```python
from build123d import *

# Parameters (mm, degrees)
BOX018_W     = 3.1
BOX018_H     = 1.2
BOX018_DEPTH = 0.2
BOX017_W     = 0.6
BOX017_H     = 1.1
BOX017_DEPTH = 0.2
BOX016_W     = 0.6
BOX016_H     = 1.1
BOX016_DEPTH = 0.2
BOX015_W     = 0.6
BOX015_H     = 1.1
BOX015_DEPTH = 0.2
BOX014_W     = 0.6
BOX014_H     = 1.1
BOX014_DEPTH = 0.2
BOX019_W     = 7.2
BOX019_H     = 3.5
BOX019_DEPTH = 0.2


with BuildPart() as cube018:
    # Box018 → Box018 (new body)
    with BuildSketch(Plane(origin=(2.05, 0, 1.3), x_dir=(1, 0, 0), z_dir=(0, 0, 1))):
        with Locations((1.55, 0.6)):
            Rectangle(BOX018_W, BOX018_H)
    extrude(amount=BOX018_DEPTH)


with BuildPart() as cube017:
    # Box017 → Box017 (new body)
    with BuildSketch(Plane(origin=(0, 2.4, 1.3), x_dir=(1, 0, 0), z_dir=(0, 0, 1))):
        with Locations((0.3, 0.55)):
            Rectangle(BOX017_W, BOX017_H)
    extrude(amount=BOX017_DEPTH)


with BuildPart() as cube016:
    # Box016 → Box016 (new body)
    with BuildSketch(Plane.XY.offset(1.3)):
        with Locations((0.3, 0.55)):
            Rectangle(BOX016_W, BOX016_H)
    extrude(amount=BOX016_DEPTH)


with BuildPart() as cube015:
    # Box015 → Box015 (new body)
    with BuildSketch(Plane(origin=(6.6, 2.4, 1.3), x_dir=(1, 0, 0), z_dir=(0, 0, 1))):
        with Locations((0.3, 0.55)):
            Rectangle(BOX015_W, BOX015_H)
    extrude(amount=BOX015_DEPTH)


with BuildPart() as cube014:
    # Box014 → Box014 (new body)
    with BuildSketch(Plane(origin=(6.6, 0, 1.3), x_dir=(1, 0, 0), z_dir=(0, 0, 1))):
        with Locations((0.3, 0.55)):
            Rectangle(BOX014_W, BOX014_H)
    extrude(amount=BOX014_DEPTH)


with BuildPart() as silver_top:
    # Box019 → Box019 (new body)
    with BuildSketch(Plane.XY.offset(1.3)):
        with Locations((3.6, 1.75)):
            Rectangle(BOX019_W, BOX019_H)
    extrude(amount=BOX019_DEPTH)

    # Cut: cut Cube014
    add(cube014.part, mode=Mode.SUBTRACT)

    # Cut001: cut Cube015
    add(cube015.part, mode=Mode.SUBTRACT)

    # Cut002: cut Cube016
    add(cube016.part, mode=Mode.SUBTRACT)

    # Cut003: cut Cube017
    add(cube017.part, mode=Mode.SUBTRACT)

    # Cut004: cut Cube018
    add(cube018.part, mode=Mode.SUBTRACT)


solid = silver_top.part
```
Check sheet for the modelled part. Datum: model origin and axes. Units: mm. Round coordinates to 2 decimals unless told otherwise and drop trailing zeros. Loops run counter-clockwise (first coordinate to the right, second up) from the corner with the lowest first, then second, coordinate; pieces in that order, holes last. Notation, with made-up numbers: (-40, -21) -> (2, -21) arc R20 cw to (2, -17) -> close; hole circle Ø2 at (-3, 10). An arc over 180 degrees is marked (long way). Write item = value, one per line. Start each with the question number.
1) Sectioned sample at C-C, the plane x = 4.5. Record the cut outline in (y, z), plus the area to 3 significant figures.
2) Sectioned sample at B-B, the plane y = 3.25. Record the cut outline in (x, z).
3) Thickness scan on probe 1 along X at (y, z) = (0.45, 1.45); probe 2 along Y at (x, z) = (0.5, 1.4); probe 3 along X at (y, z) = (2.7, 1.4). Record the ranges inside material, lowest first.
4) Sectioned sample at A-A, the plane z = 1.4. Record the cut outline in (x, y).
Results are:
q1.outline = (1.2, 1.3) -> (3.5, 1.3) -> (3.5, 1.5) -> (1.2, 1.5) -> close
q1.area = 0.460 mm^2
q2.outline = (0.6, 1.3) -> (6.6, 1.3) -> (6.6, 1.5) -> (0.6, 1.5) -> close
q3.probe_1 = 0.6 to 2.05, 5.15 to 6.6
q3.probe_2 = 1.1 to 2.4
q3.probe_3 = 0.6 to 6.6
q4.outline = (0, 1.1) -> (0.6, 1.1) -> (0.6, 0) -> (2.05, 0) -> (2.05, 1.2) -> (5.15, 1.2) -> (5.15, 0) -> (6.6, 0) -> (6.6, 1.1) -> (7.2, 1.1) -> (7.2, 2.4) -> (6.6, 2.4) -> (6.6, 3.5) -> (0.6, 3.5) -> (0.6, 2.4) -> (0, 2.4) -> close
